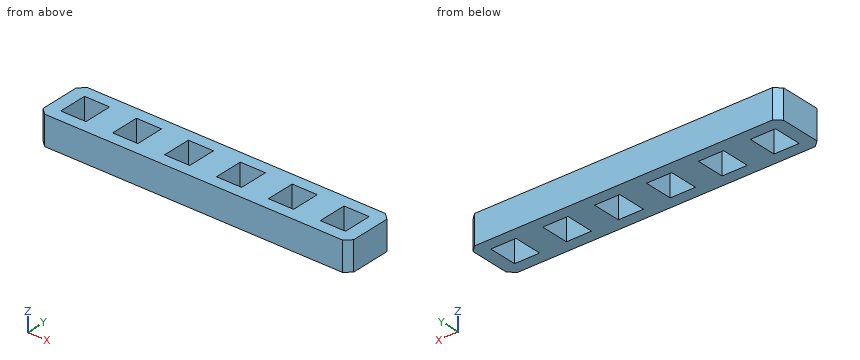
```python
from build123d import *

# Parameters (mm, degrees)
SCHIZZO1_W                   = 4.85
SCHIZZO1_H                   = 5.525
ESTRUSIONE_ESTRUSIONE2_DEPTH = 5.6


with BuildPart() as part:
    # Schizzo1 → Estrusione-Estrusione2 (new body)
    with BuildSketch(Plane.XY):
        Polygon((-30.55, 3.88125), (-30.55, -3.88125), (-29.3, -5), (28.05, -5), (29.3, -3.88125), (29.3, 3.88125), (28.05, 5), (-29.3, 5), align=None)
        with Locations((-15.625, 0)):
            Rectangle(SCHIZZO1_W, SCHIZZO1_H, mode=Mode.SUBTRACT)
        with Locations((-25.625, 0)):
            Rectangle(SCHIZZO1_W, SCHIZZO1_H, mode=Mode.SUBTRACT)
        with Locations((-5.625, 0)):
            Rectangle(SCHIZZO1_W, SCHIZZO1_H, mode=Mode.SUBTRACT)
        with Locations((4.375, 0)):
            Rectangle(SCHIZZO1_W, SCHIZZO1_H, mode=Mode.SUBTRACT)
        with Locations((14.375, 0)):
            Rectangle(SCHIZZO1_W, SCHIZZO1_H, mode=Mode.SUBTRACT)
        with Locations((24.375, 0)):
            Rectangle(SCHIZZO1_W, SCHIZZO1_H, mode=Mode.SUBTRACT)
    extrude(amount=ESTRUSIONE_ESTRUSIONE2_DEPTH)


solid = part.part
```
Part model, mm, in its own coordinate system. Round coordinates to 2 decimals unless told otherwise and drop trailing zeros. Write each loop counter-clockwise with the first axis right and the second up, starting at its lowest first coordinate (ties: lowest second). Pieces come first, ordered by that corner, then holes.
Item 1: Cut at A-A, the plane y = -1.5. Give the cut face in (x, z).
Results:
outline: (-30.55, 0) - (-28.05, 0) - (-28.05, 5.6) - (-30.55, 5.6) - close; (-23.2, 0) - (-18.05, 0) - (-18.05, 5.6) - (-23.2, 5.6) - close; (-13.2, 0) - (-8.05, 0) - (-8.05, 5.6) - (-13.2, 5.6) - close; (-3.2, 0) - (1.95, 0) - (1.95, 5.6) - (-3.2, 5.6) - close; (6.8, 0) - (11.95, 0) - (11.95, 5.6) - (6.8, 5.6) - close; (16.8, 0) - (21.95, 0) - (21.95, 5.6) - (16.8, 5.6) - close; (26.8, 0) - (29.3, 0) - (29.3, 5.6) - (26.8, 5.6) - close
Item 2: Drop a flat-ended pin along its axis: pin 1 Ø2 at (y, z) = (-4, 4.5) entering from -X. Give the stop position or say it passes through.
Results:
pin 1: stops at x = -30.55
Item 3: Cut at B-B, the plane z = 2.8. Count the separate pieces of the cut face and the enclosed holes in it, plus the area to 3 significant figures.
Results:
separate pieces: 1
enclosed holes: 6
area: 435 mm2
Item 4: Probe L1, parallel to Y at x = 15, z = 2.85; L2, parallel to X at y = -4.5, z = 0.65; L3, parallel to X at y = -4.25, z = 4.2. List the from-to ranges inside material, lowest first.
Results:
L1: y = -5 to -2.76, 2.76 to 5
L2: x = -29.86 to 28.61
L3: x = -30.14 to 28.89
Item 5: Cut at C-C, the plane x = -7. Give the cut face in (y, z), plus the area to 3 significant figures.
Results:
outline: (-5, 0) - (-2.76, 0) - (-2.76, 5.6) - (-5, 5.6) - close; (2.76, 0) - (5, 0) - (5, 5.6) - (2.76, 5.6) - close
area: 25.1 mm2
